from build123d import *

# Parameters (mm, degrees)
SKETCH_1_W          = 15
SKETCH_1_H          = 15
SKETCH_1_W_2        = 13
SKETCH_1_H_2        = 13
EXTRUDE_1_DEPTH     = 460
SKETCH_2_R          = 1.45
CUT_EXTRUDE_1_DEPTH = 461.305605006
SKETCH_3_R          = 1.45
CUT_EXTRUDE_2_DEPTH = 461.305605006


with BuildPart() as part:
    # 草图1 → 拉伸-薄壁1 (new body)
    with BuildSketch(Plane(origin=(0, 0, 0), x_dir=(1, 0, 0), z_dir=(0, 1, 0))):
        Rectangle(SKETCH_1_W, SKETCH_1_H)
        Rectangle(SKETCH_1_W_2, SKETCH_1_H_2, mode=Mode.SUBTRACT)
    extrude(amount=EXTRUDE_1_DEPTH)

    # 草图2 → 切除-拉伸1 (cut, through all)
    with BuildSketch(Plane.XY.offset(7.5)):
        with Locations((0, 7.5)):
            Circle(SKETCH_2_R)
        with Locations((0, 27.5)):
            Circle(SKETCH_2_R)
        with Locations(Location((0, 432.5, 0), (0, 0, 180))):
            Circle(SKETCH_2_R)
        with Locations(Location((0, 452.5, 0), (0, 0, 180))):
            Circle(SKETCH_2_R)
        with Locations((0, 140)):
            Circle(SKETCH_2_R)
        with Locations((0, 160)):
            Circle(SKETCH_2_R)
        with Locations((0, 120)):
            Circle(SKETCH_2_R)
        with Locations(Location((0, 340, 0), (0, 0, 180))):
            Circle(SKETCH_2_R)
        with Locations(Location((0, 300, 0), (0, 0, 180))):
            Circle(SKETCH_2_R)
        with Locations(Location((0, 320, 0), (0, 0, 180))):
            Circle(SKETCH_2_R)
        with Locations((0, 230)):
            Circle(SKETCH_2_R)
        with Locations((0, 255)):
            Circle(SKETCH_2_R)
        with Locations((0, 205)):
            Circle(SKETCH_2_R)
        with Locations((0, 95)):
            Circle(SKETCH_2_R)
        with Locations(Location((0, 365, 0), (0, 0, 180))):
            Circle(SKETCH_2_R)
        with Locations((0, 75)):
            Circle(SKETCH_2_R)
        with Locations(Location((0, 385, 0), (0, 0, 180))):
            Circle(SKETCH_2_R)
    extrude(amount=-CUT_EXTRUDE_1_DEPTH, mode=Mode.SUBTRACT)

    # 草图3 → 切除-拉伸2 (cut, through all)
    with BuildSketch(Plane(origin=(7.5, 0, 0), x_dir=(0, 0, -1), z_dir=(1, 0, 0))):
        with Locations((0, 15)):
            Circle(SKETCH_3_R)
        with Locations((0, 35)):
            Circle(SKETCH_3_R)
        with Locations((0, 425)):
            Circle(SKETCH_3_R)
        with Locations((0, 445)):
            Circle(SKETCH_3_R)
        with Locations((0, 172.5)):
            Circle(SKETCH_3_R)
        with Locations((0, 192.5)):
            Circle(SKETCH_3_R)
        with Locations((0, 152.5)):
            Circle(SKETCH_3_R)
        with Locations((0, 307.5)):
            Circle(SKETCH_3_R)
        with Locations((0, 267.5)):
            Circle(SKETCH_3_R)
        with Locations((0, 287.5)):
            Circle(SKETCH_3_R)
        with Locations((0, 55)):
            Circle(SKETCH_3_R)
        with Locations((0, 405)):
            Circle(SKETCH_3_R)
    extrude(amount=-CUT_EXTRUDE_2_DEPTH, mode=Mode.SUBTRACT)


solid = part.part
Geometry: final body of the model. Coordinates: model frame, mm. A direction names the side the tool comes from. Give positions to 0.01 mm unless a question says otherwise; leave off trailing zeros. Write each loop counter-clockwise with the first axis right and the second up, starting at its lowest first coordinate (ties: lowest second). Pieces come first, ordered by that corner, then holes.
(1) Access query for faces 1 (the flat face through (-6.5, 227, 0)), 2 (the flat face through (7.5, 227, 0)). Directions: +Z, -Z, +X, -X, +Y, -Y. A direction counts if a zero-diameter tool reaches every point of the face in a straight line with its end or side. Return the directions, or none.
(2) Cut plane B-B, the plane y = 332.5. Return loops of the section in (x, z), then the cut area to 3 significant figures.
(3) Cut plane A-A, the plane z = 4.25. Return loops of the section in (x, y), then the cut area to 3 significant figures.
(4) Cut plane C-C, the plane x = -4. Return loops of the section in (y, z), then the cut area to 3 significant figures.
(5) Mould query, pull axis X, two halves, no side actions, for faces 3 (the flat face through (-7.5, 227, 0)), 4 (the flat face through (6.5, 227, 0)), 5 (the flat face through (0, 227, -7.5)). Classes: released by +X, released by -X, zero draft, split by the parting line, or undercut.
(6) Ray query, line 1 (X direction, y = 108, z = -3.5); line 2 (Z direction, x = 7.05, y = 307.5). Return the intervals inside material, ascending.
(7) First-contact query: P1, Ø1.7, axis at x = 0, y = 95, coming from the +Z side. Flat tip, straight axial feed; report the tip coordinate or a pass-through.
Values follow:
1. face 1: +Y, -Y
1. face 2: +Z, -Z, +X, +Y, -Y
2. outline: (-7.5, -7.5) - (7.5, -7.5) - (7.5, 7.5) - (-7.5, 7.5) - close; hole (-6.5, -6.5) - (6.5, -6.5) - (6.5, 6.5) - (-6.5, 6.5) - close
2. area: 56.0 mm2
3. outline: (-7.5, 0) - (-6.5, 0) - (-6.5, 460) - (-7.5, 460) - close; (6.5, 0) - (7.5, 0) - (7.5, 460) - (6.5, 460) - close
3. area: 920 mm2
4. outline: (0, -7.5) - (460, -7.5) - (460, -6.5) - (0, -6.5) - close; (0, 6.5) - (460, 6.5) - (460, 7.5) - (0, 7.5) - close
4. area: 920 mm2
5. face 3: released by -X
5. face 4: undercut
5. face 5: zero draft
6. line 1: x = -7.5 to -6.5, 6.5 to 7.5
6. line 2: z = -7.5 to -1.45, 1.45 to 7.5
7. P1: passes through
